For this review, use the dimensioned drawing (mm, ordinates from the lowest corner) and the shaded views. Round coordinates to 2 decimals unless told otherwise and drop trailing zeros. Write each loop counter-clockwise with the first axis right and the second up, starting at its lowest first coordinate (ties: lowest second). Pieces come first, ordered by that corner, then holes. Notation, with made-up numbers: M 49,4.5 L 88,4.5 A30 cw 88,30.5 Z; hole C 68,-7 d3. An arc over 180 degrees is marked long. Use CSV: the item, a comma, the result in double quotes.
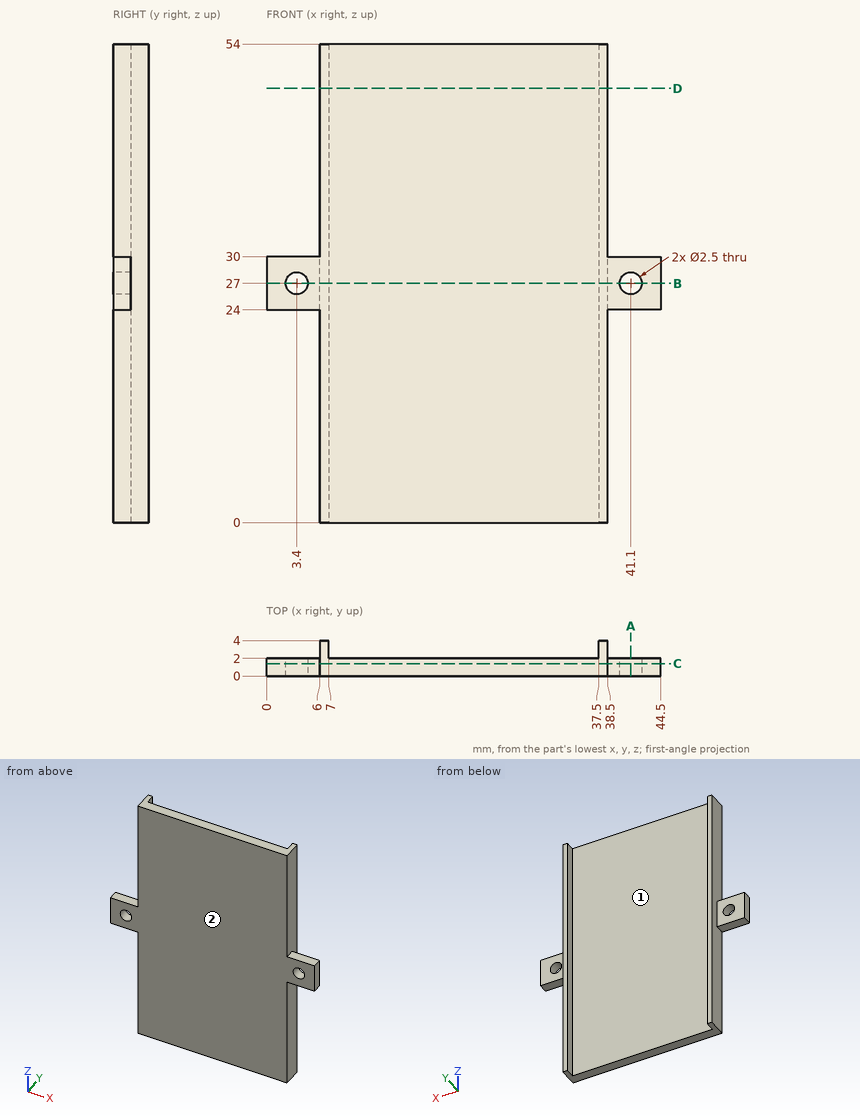
1) For pin 1 Ø1.5 at (x, y) = (18, 2.5) entering from -Z; pin 2 Ø1.5 at (x, z) = (21, 8) entering from +Y; pin 3 Ø2 at (x, y) = (42.5, 0.5) entering from +Z; pin 4 Ø2 at (y, z) = (2.5, 15.5) entering from +X, all flat-tipped, find the tip position at first contact; note any pin that passes through.
Answers:
pin 1,"z = 0"
pin 2,"y = 2"
pin 3,"z = 30"
pin 4,"x = 38.5"
2) Add section D-D on z = 49. Write out the cut boundary in (x, y).
Answers:
outline,"M 6,0 L 38.5,0 L 38.5,4 L 37.5,4 L 37.5,2 L 7,2 L 7,4 L 6,4 Z"
3) Wall thickness on line 1 along X through (y, z) = (1.8, 26); line 2 along Z through (x, y) = (3.4, 0.75); line 3 along Y through (x, z) = (20, 25): over which ranges is each line inside the solid? List them lowest first. Write a range as [from, to].
Answers:
line 1,"[0, 2.65], [4.15, 40.35], [41.85, 44.5]"
line 2,"[24, 25.75], [28.25, 30]"
line 3,"[0, 2]"
4) The part is to be moulded in two halves that separate along X. For the marked faces 1 and 2, say which applies: released by +X, released by -X, zero draft, split by the parting line, or undercut.
Answers:
face 1,"undercut"
face 2,"zero draft"
5) Add section B-B on z = 27. Write out the cut boundary in (x, y).
Answers:
outline,"M 0,0 L 2.15,0 L 2.15,2 L 0,2 Z; M 4.65,0 L 39.85,0 L 39.85,2 L 38.5,2 L 38.5,4 L 37.5,4 L 37.5,2 L 7,2 L 7,4 L 6,4 L 6,2 L 4.65,2 Z; M 42.35,0 L 44.5,0 L 44.5,2 L 42.35,2 Z"
6) Add section A-A on x = 41.1. Write out the cut boundary in (y, z).
Answers:
outline,"M 0,24 L 2,24 L 2,25.75 L 0,25.75 Z; M 0,28.25 L 2,28.25 L 2,30 L 0,30 Z"
7) Add section C-C on y = 1.4. Write out the cut boundary in (x, z), then the cut area to 3 significant figures.
Answers:
outline,"M 0,24 L 6,24 L 6,0 L 38.5,0 L 38.5,24 L 44.5,24 L 44.5,30 L 38.5,30 L 38.5,54 L 6,54 L 6,30 L 0,30 Z; hole C 3.4,27 d2.5; hole C 41.1,27 d2.5"
area,"1,820 mm²"
